Check sheet for the modelled part. Datum: model origin and axes. Units: mm. A direction names the side the tool comes from. Coordinates: 2 decimals unless noted, no trailing zeros. Loops run counter-clockwise (first coordinate to the right, second up) from the corner with the lowest first, then second, coordinate; pieces in that order, holes last. Notation, with made-up numbers: M -11,33.5 L 13,33.5 A36 ccw 13,67.5 Z; hole C -13.75,51.25 d7. An arc over 180 degrees is marked long. Answer as CSV lines item,"result". Start each with the question number.
from build123d import *

# Parameters (mm, degrees)
F0_R      = 18
F1_DEPTH  = 8
F2_R      = 18
F2_R_2    = 11.875
F3_DEPTH  = 96
F7_W      = 114.2527745105
F7_H      = 71.0478108376
F8_DEPTH  = 19
F9_W      = 142.8963663056
F9_H      = 89.3513672054
F10_DEPTH = 19
F12_DEPTH = 104
F14_W     = 80
F14_H     = 12.8310857864
F15_DEPTH = 3.5
F16_W     = 12.3001844622
F16_H     = 37.9971187711
F16_H_2   = 3.5
F17_DEPTH = 2
F18_W     = 82.2026617825
F18_H     = 23.6075371504
F19_DEPTH = 2
F22_DEPTH = 13.5
F24_W     = 39.2900933512
F24_H     = 12.6941720955
F25_DEPTH = 1.3
F26_DEPTH = 2.4


with BuildPart() as f1:
    # F0 (on Top) → F1 (new body)
    with BuildSketch(Plane.XY):
        with Locations((-64.5627826452, 2.4795725476)):
            Circle(F0_R)
    extrude(amount=F1_DEPTH)

    # F2 (on face) → F3 (join)
    with BuildSketch(Plane.XY.offset(8)):
        with Locations((-64.5627826452, 2.4795725476)):
            Circle(F2_R)
        with Locations((-64.5627826452, 2.4795725476)):
            Circle(F2_R_2, mode=Mode.SUBTRACT)
    extrude(amount=F3_DEPTH)

    # F7 (on offset) → F8 (cut)
    with BuildSketch(Plane.XY.offset(66)):
        with Locations((-59.9692843389, 7.8492248431)):
            Rectangle(F7_W, F7_H)
    extrude(amount=F8_DEPTH, mode=Mode.SUBTRACT)

    # F9 (on offset) → F10 (cut)
    with BuildSketch(Plane.XY.offset(47)):
        with Locations((-63.3265613578, 3.715576604)):
            Rectangle(F9_W, F9_H)
    extrude(amount=-F10_DEPTH, mode=Mode.SUBTRACT)

    # F11 (on Top) → F12 (join)
    with BuildSketch(Plane.XY):
        Polygon((-46.4286282659, 8.8664737705), (-47.033398658, 8.8664737705), (-49.5477505028, 8.8664737705), (-49.5477505028, -3.6335218174), (-47.033398658, -3.6335218174), (-46.4286282659, -3.6335218174), align=None)
    extrude(amount=F12_DEPTH)

    # F14 (on offset) → F15 (join)
    with BuildSketch(Plane.XY.offset(66)):
        with Locations((-7.5557883829, 2.6472329628)):
            Rectangle(F14_W, F14_H)
    extrude(amount=-F15_DEPTH)

    # F16 (on face) → F17 (join)
    with BuildSketch(Plane.YZ.offset(32.4442116171)):
        with Locations((2.3817823007, 84.9985593855)):
            Rectangle(F16_W, F16_H)
        with Locations((2.3817823007, 64.25)):
            Rectangle(F16_W, F16_H_2)
    extrude(amount=F17_DEPTH)

    # F18 (on face) → F19 (join)
    with BuildSketch(Plane.XZ.offset(3.6335218174)):
        with Locations((-6.6709686071, 92.0722857118)):
            Rectangle(F18_W, F18_H)
    extrude(amount=F19_DEPTH)

    # F21 (on offset) → F22 (join)
    with BuildSketch(Plane.XY.offset(62.6)):
        with BuildLine():
            Line((31.0583338141, 8.7254531682), (32.4985198677, 8.7659778073))
            ThreePointArc((32.4985198677, 8.7659778073), (-7.1450361543, 16.8829381262), (-46.6268882155, 8.0127669498))
            Line((-46.6268882155, 8.0127669498), (-45.5970168114, 7.9405866563))
            ThreePointArc((-45.5970168114, 7.9405866563), (-7.3488744174, 16.1007405169), (31.0583338141, 8.7254531682))
        make_face()
    extrude(amount=F22_DEPTH)



with BuildPart() as f25:
    # F24 (on offset) → F25 (new body)
    with BuildSketch(Plane.XY.offset(33.6)):
        with Locations((-26.6252344009, 2.7435675729)):
            Rectangle(F24_W, F24_H)
    extrude(amount=-F25_DEPTH)


with BuildPart() as f1_1:
    add(f1.part)
    # F26 (add): a face of the model
    f26_faces = [f25.part.faces().sort_by_distance(p)[0] for p in [
        (-46.2702810764, 2.7435675729, 32.95),
    ]]

    add(f25.part)  # F26 merges F25
    extrude(f26_faces, amount=F26_DEPTH)


solid = f1_1.part
Item 1: Material ranges on line 1 (Z direction, x = -50.5, y = -7); line 2 (Z direction, x = -9.5, y = 5); line 3 (X direction, y = 6, z = 78), recorded low to high. Write a range as from..to.
Item 2: Sectioned sample at C-C, the plane y = -7. Record the boundary of the cut face in (x, z).
Item 3: Sectioned sample at D-D, the plane y = 11.5. Give the number of separate pieces and of enclosed holes in the cut face, and give its area (3 significant figures).
Item 4: Release check for a two-part mould opening along Z. For faces 1 (the face through (-49.548, 3, 75)), 2 (the face through (34.444, 2, 84)), 3 (the face through (-7.1, 16.4, 76.1)) record: released by +Z, released by -Z, zero draft, split by the parting line, or undercut.
Item 5: Sectioned sample at A-A, the plane x = -74.5. Record the boundary of the cut face in (y, z).
Item 6: Go/stop test with flat-tipped pins: pin 1 (10.5 mm diameter, centred on x = 10.5, y = 0, fed in from +Z); pin 2 (3 mm diameter, centred on x = 6.5, y = 16.5, fed in from +Z); pin 3 (2 mm diameter, centred on x = -3.5, y = -2.5, fed in from -Z); pin 4 (10 mm diameter, centred on y = 1.5, z = 88, fed in from -X). Record where each tip stops, or that it passes through.
Item 7: Set-up check for faces 4 (the face through (-49.548, 3, 37)), 5 (the face through (-1, -3.768, 65)), 6 (the face through (-7, 3, 62.5)), 7 (the face through (-60.7, -9.3, 104)): record each of +Z, -Z, +X, -X, +Y, -Y from which the full face is reachable in a straight line by a thin tool's end or side.
Reply:
1,line 1,"0..28, 47..66, 85..104"
1,line 2,"32.3..33.6, 62.5..66"
1,line 3,"-49.55..-46.43, 32.44..34.44"
2,outline,"M -79.86,0 L -49.26,0 L -49.26,28 L -57.41,28 L -57.41,8 L -71.71,8 L -71.71,28 L -79.86,28 Z; M -79.86,47 L -71.71,47 L -71.71,66 L -79.86,66 Z; M -79.86,85 L -71.71,85 L -71.71,104 L -79.86,104 Z; M -57.41,47 L -49.26,47 L -49.26,66 L -57.41,66 Z; M -57.41,85 L -49.26,85 L -49.26,104 L -57.41,104 Z"
3,separate pieces,"7"
3,enclosed holes,"0"
3,area,"1,210 mm²"
4,face 1,"undercut"
4,face 2,"zero draft"
4,face 3,"released by +Z"
5,outline,"M -12.53,0 L 17.49,0 L 17.49,28 L 8.98,28 L 8.98,8 L -4.02,8 L -4.02,28 L -12.53,28 Z; M -12.53,47 L -4.02,47 L -4.02,66 L -12.53,66 Z; M -12.53,85 L -4.02,85 L -4.02,104 L -12.53,104 Z; M 8.98,47 L 17.49,47 L 17.49,66 L 8.98,66 Z; M 8.98,85 L 17.49,85 L 17.49,104 L 8.98,104 Z"
6,pin 1,"z = 103.88"
6,pin 2,"z = 76.1"
6,pin 3,"z = 62.5"
6,pin 4,"x = -82.56"
7,face 4,"-X, +Y, -Y"
7,face 5,"-Z, +X, -Y"
7,face 6,"+X, +Y, -Y"
7,face 7,"+Z, +X, -X, +Y, -Y"
